from build123d import *

# Parameters (mm, degrees)
F0_W      = 120
F0_H      = 60
F0_R      = 4
F1_DEPTH  = 10
F3_W      = 90
F3_H      = 100
F4_DEPTH  = 5
F7_D      = 4.4
F8_D      = 4.4
F9_R      = 5
F10_R     = 5
F11_R     = 5
F12_R     = 5
F13_R     = 5
F14_R     = 5
F16_DEPTH = 5


# Not quite as in the source:
# - a feature of the source that left no trace in its solid (it failed there, or was rolled back) is left out


with BuildPart() as f1:
    # F0 (on Top) → F1 (new body)
    with BuildSketch(Plane.XY):
        Rectangle(F0_W, F0_H)
        with Locations((-50, 0)):
            Circle(F0_R, mode=Mode.SUBTRACT)
        with Locations((50, 0)):
            Circle(F0_R, mode=Mode.SUBTRACT)
    extrude(amount=-F1_DEPTH)

    # F3 (on offset) → F4 (join)
    with BuildSketch(Plane.XZ.offset(18)):
        with Locations((0, 50)):
            Rectangle(F3_W, F3_H)
    extrude(amount=F4_DEPTH)

    # F7 (through all)
    with Locations(Plane(origin=(0, -18, 0), x_dir=(1, 0, 0), z_dir=(0, 1, 0))):
        with Locations((20.9, -95.8)):
            Hole(F7_D / 2)

    # F8 (through all)
    with Locations(Plane(origin=(0, -18, 0), x_dir=(1, 0, 0), z_dir=(0, 1, 0))):
        with Locations((20.9, -27.8)):
            Hole(F8_D / 2)

    # F9
    f9_edges = [f1.edges().sort_by_distance(p)[0] for p in [
        (-60, -30, -5),
    ]]
    fillet(f9_edges, radius=F9_R)

    # F10
    f10_edges = [f1.edges().sort_by_distance(p)[0] for p in [
        (-60, 30, -5),
    ]]
    fillet(f10_edges, radius=F10_R)

    # F11
    f11_edges = [f1.edges().sort_by_distance(p)[0] for p in [
        (60, 30, -5),
    ]]
    fillet(f11_edges, radius=F11_R)

    # F12
    f12_edges = [f1.edges().sort_by_distance(p)[0] for p in [
        (60, -30, -5),
    ]]
    fillet(f12_edges, radius=F12_R)

    # F13
    f13_edges = [f1.edges().sort_by_distance(p)[0] for p in [
        (45, -20.5, 100),
    ]]
    fillet(f13_edges, radius=F13_R)

    # F14
    f14_edges = [f1.edges().sort_by_distance(p)[0] for p in [
        (-45, -20.5, 100),
    ]]
    fillet(f14_edges, radius=F14_R)

    # F15 (on Right) → F16 (join, symmetric)
    with BuildSketch(Plane.YZ):
        Polygon((0, 0), (-18, 15), (-18, 0), align=None)
    extrude(amount=F16_DEPTH, both=True)


solid = f1.part
Here's how the part is built. I have some questions about the finished solid (model axes, mm). A direction names the side the tool comes from. Round coordinates to 2 decimals unless told otherwise and drop trailing zeros. Order: outer loops, then holes, each group sorted by start corner. A loop starts at its lowest first (then second) coordinate and runs counter-clockwise, first axis right, second up. Notation, with made-up numbers: M 75.25,0.25 L 86.25,0.25 A18 ccw 86.25,32.25 Z; hole C 70.5,57.25 d3. An arc over 180 degrees is marked long. Return JSON: item names as keys, results as strings. Group by question number.
1. If we section it at D-D on z = 7.5: List the corners of the cut face in (x, y) for me, then the cut area to 3 significant figures.
2. If we section it at A-A on z = 27.8: List the corners of the cut face in (x, y) for me, then the cut area to 3 significant figures.
3. Please list where these lines run through material, in increasing order: probe 1 along Z at (x, y) = (20.9, -21.15); probe 2 along Y at (x, z) = (50, -7); probe 3 along Z at (x, y) = (51, -8.5).
4. If we mould it in two halves opening along X, with no side actions, what happens to faces 4 (the face through (46, 0, -5)), 5 (the face through (-60, 0, -5)), 6 (the face through (60, 0, -5))? For each: pulls with the +X half, pulls with the -X half, needs draft (parallel to the pull), parting line crosses it, or undercut.
5. If we section it at C-C on x = 20.9: List the corners of the cut face in (y, z) for me, then the cut area to 3 significant figures.
6. On a 3-axis mill with a long thin cutter (end or side, diameter ignored), from which of +Z, -Z, +X, -X, +Y, -Y can I reach the whole of each face in a straight line? I mean faces 1 (the face through (45, -20, 47)), 2 (the face through (5, -13, 4)), 3 (the face through (-45, -20, 47)). Say none if no direction works.
7. I'm going to push flat-ended pins straight in: pin 1 Ø6 at (x, z) = (-47.5, 4) entering from +Y; pin 2 Ø12 at (x, z) = (-7, 75.5) entering from -Y; pin 3 Ø6 at (x, y) = (39.5, 2.5) entering from +Z. Where does each tip first touch, or does it pass through?
8. If we section it at B-B on x = 50: List the corners of the cut face in (y, z) for me, then the cut area to 3 significant figures.
Reply:
{
 "1": {"outline": "M -45,-23 L 45,-23 L 45,-18 L 5,-18 L 5,-9 L -5,-9 L -5,-18 L -45,-18 Z", "area": "540 mm^2"},
 "2": {"outline": "M -45,-23 L 18.7,-23 L 18.7,-18 L -45,-18 Z; M 23.1,-23 L 45,-23 L 45,-18 L 23.1,-18 Z", "area": "428 mm^2"},
 "3": {"probe 1": "-10 to 25.6, 30 to 93.6, 98 to 100", "probe 2": "-30 to -4, 4 to 30", "probe 3": "-10 to 0"},
 "4": {"face 4": "undercut", "face 5": "pulls with the -X half", "face 6": "pulls with the +X half"},
 "5": {"outline": "M -30,-10 L 30,-10 L 30,0 L -18,0 L -18,25.6 L -23,25.6 L -23,0 L -30,0 Z; M -23,30 L -18,30 L -18,93.6 L -23,93.6 Z; M -23,98 L -18,98 L -18,100 L -23,100 Z", "area": "1,060 mm^2"},
 "6": {"face 1": "+Z, +X, +Y, -Y", "face 2": "+Z, +X, +Y", "face 3": "+Z, -X, +Y, -Y"},
 "7": {"pin 1": "y = -18", "pin 2": "y = -23", "pin 3": "z = 0"},
 "8": {"outline": "M -30,-10 L -4,-10 L -4,0 L -30,0 Z; M 4,-10 L 30,-10 L 30,0 L 4,0 Z", "area": "520 mm^2"}
}
